Part model, mm, in its own coordinate system. A direction names the side the tool comes from. Round coordinates to 2 decimals unless told otherwise and drop trailing zeros. Order: outer loops, then holes, each group sorted by start corner. A loop starts at its lowest first (then second) coordinate and runs counter-clockwise, first axis right, second up. Notation, with made-up numbers: (74, 46) - (93, 46) arc R19 cw to (93, 62) - close; hole circle Ø1 at (-30.5, 86). An arc over 180 degrees is marked (long way). Return JSON: item names as keys, results as strings. Group by question number.
Item 1: Saw through at A-A on y = 0. List the corners of the cut face in (x, z).
Item 2: Probe probe 1 along Y at (x, z) = (7.5, 36); probe 2 along X at (y, z) = (7, 61); probe 3 along Y at (x, z) = (0, 69). List the from-to ranges inside material, lowest first.
Item 3: Drop flat-ended pins along their axis: pin 1 (5 mm diameter, centred on x = 0, z = 50, fed in from +Y); pin 2 (2.5 mm diameter, centred on y = 0, z = 31.5, fed in from +X). Give the stop position or say it passes through.
Item 4: Two-plate mould, pull along Y, no slides. Class faces 5 (the face through (-2, 2, 0)), 6 (the face through (6, -10, 49)), 7 (the face through (-8, 4, 49)): released by +Y, released by -Y, zero draft, split by the parting line, or undercut.
Item 5: Tool access for faces 1 (the face through (-4, 0, 49)), 2 (the face through (10, 6, 49)), 3 (the face through (0, 4, 49)), 4 (the face through (5, -8, 49)): list every direction of +Z, -Z, +X, -X, +Y, -Y with a clear straight run to the whole face (end or side of a thin tool).
```python
from build123d import *

# Parameters (mm, degrees)
SKETCH2_R           = 2.5
BOSS_EXTRUDE1_DEPTH = 100


with BuildPart() as part:
    # Sketch2 → Boss-Extrude1 (new body)
    with BuildSketch(Plane.XY):
        with BuildLine():
            Line((10, 3.25), (10, 9))
            ThreePointArc((10, 9), (9.707106781, 9.707106781), (9, 10))
            Line((9, 10), (3.25, 10))
            ThreePointArc((3.25, 10), (3.073223305, 9.926776695), (3, 9.75))
            Line((3, 9.75), (3, 8.25))
            ThreePointArc((3, 8.25), (3.073223305, 8.073223305), (3.25, 8))
            Line((3.25, 8), (5.75, 8))
            ThreePointArc((5.75, 8), (5.926776695, 7.926776695), (6, 7.75))
            Line((6, 7.75), (6, 7.164213562))
            ThreePointArc((6, 7.164213562), (5.980969883, 7.068542704), (5.926776695, 6.987436867))
            Line((5.926776695, 6.987436867), (3.085786438, 4.146446609))
            ThreePointArc((3.085786438, 4.146446609), (2.923574763, 4.038060234), (2.732233047, 4))
            Line((2.732233047, 4), (-2.732233047, 4))
            ThreePointArc((-2.732233047, 4), (-2.923574763, 4.038060234), (-3.085786438, 4.146446609))
            Line((-3.085786438, 4.146446609), (-5.926776695, 6.987436867))
            ThreePointArc((-5.926776695, 6.987436867), (-5.980969883, 7.068542704), (-6, 7.164213562))
            Line((-6, 7.164213562), (-6, 7.75))
            ThreePointArc((-6, 7.75), (-5.926776695, 7.926776695), (-5.75, 8))
            Line((-5.75, 8), (-3.25, 8))
            ThreePointArc((-3.25, 8), (-3.073223305, 8.073223305), (-3, 8.25))
            Line((-3, 8.25), (-3, 9.75))
            ThreePointArc((-3, 9.75), (-3.073223305, 9.926776695), (-3.25, 10))
            Line((-3.25, 10), (-9, 10))
            ThreePointArc((-9, 10), (-9.707106781, 9.707106781), (-10, 9))
            Line((-10, 9), (-10, 3.25))
            ThreePointArc((-10, 3.25), (-9.926776695, 3.073223305), (-9.75, 3))
            Line((-9.75, 3), (-8.25, 3))
            ThreePointArc((-8.25, 3), (-8.073223305, 3.073223305), (-8, 3.25))
            Line((-8, 3.25), (-8, 5.75))
            ThreePointArc((-8, 5.75), (-7.926776695, 5.926776695), (-7.75, 6))
            Line((-7.75, 6), (-7.164213562, 6))
            ThreePointArc((-7.164213562, 6), (-7.068542704, 5.980969883), (-6.987436867, 5.926776695))
            Line((-6.987436867, 5.926776695), (-4.146446609, 3.085786438))
            ThreePointArc((-4.146446609, 3.085786438), (-4.038060234, 2.923574763), (-4, 2.732233047))
            Line((-4, 2.732233047), (-4, -2.732233047))
            ThreePointArc((-4, -2.732233047), (-4.038060234, -2.923574763), (-4.146446609, -3.085786438))
            Line((-4.146446609, -3.085786438), (-6.987436867, -5.926776695))
            ThreePointArc((-6.987436867, -5.926776695), (-7.068542704, -5.980969883), (-7.164213562, -6))
            Line((-7.164213562, -6), (-7.75, -6))
            ThreePointArc((-7.75, -6), (-7.926776695, -5.926776695), (-8, -5.75))
            Line((-8, -5.75), (-8, -3.25))
            ThreePointArc((-8, -3.25), (-8.073223305, -3.073223305), (-8.25, -3))
            Line((-8.25, -3), (-9.75, -3))
            ThreePointArc((-9.75, -3), (-9.926776695, -3.073223305), (-10, -3.25))
            Line((-10, -3.25), (-10, -9))
            ThreePointArc((-10, -9), (-9.707106781, -9.707106781), (-9, -10))
            Line((-9, -10), (-3.25, -10))
            ThreePointArc((-3.25, -10), (-3.073223305, -9.926776695), (-3, -9.75))
            Line((-3, -9.75), (-3, -8.25))
            ThreePointArc((-3, -8.25), (-3.073223305, -8.073223305), (-3.25, -8))
            Line((-3.25, -8), (-5.75, -8))
            ThreePointArc((-5.75, -8), (-5.926776695, -7.926776695), (-6, -7.75))
            Line((-6, -7.75), (-6, -7.164213562))
            ThreePointArc((-6, -7.164213562), (-5.980969883, -7.068542704), (-5.926776695, -6.987436867))
            Line((-5.926776695, -6.987436867), (-3.085786438, -4.146446609))
            ThreePointArc((-3.085786438, -4.146446609), (-2.923574763, -4.038060234), (-2.732233047, -4))
            Line((-2.732233047, -4), (2.732233047, -4))
            ThreePointArc((2.732233047, -4), (2.923574763, -4.038060234), (3.085786438, -4.146446609))
            Line((3.085786438, -4.146446609), (5.926776695, -6.987436867))
            ThreePointArc((5.926776695, -6.987436867), (5.980969883, -7.068542704), (6, -7.164213562))
            Line((6, -7.164213562), (6, -7.75))
            ThreePointArc((6, -7.75), (5.926776695, -7.926776695), (5.75, -8))
            Line((5.75, -8), (3.25, -8))
            ThreePointArc((3.25, -8), (3.073223305, -8.073223305), (3, -8.25))
            Line((3, -8.25), (3, -9.75))
            ThreePointArc((3, -9.75), (3.073223305, -9.926776695), (3.25, -10))
            Line((3.25, -10), (9, -10))
            ThreePointArc((9, -10), (9.707106781, -9.707106781), (10, -9))
            Line((10, -9), (10, -3.25))
            ThreePointArc((10, -3.25), (9.926776695, -3.073223305), (9.75, -3))
            Line((9.75, -3), (8.25, -3))
            ThreePointArc((8.25, -3), (8.073223305, -3.073223305), (8, -3.25))
            Line((8, -3.25), (8, -5.75))
            ThreePointArc((8, -5.75), (7.926776695, -5.926776695), (7.75, -6))
            Line((7.75, -6), (7.164213562, -6))
            ThreePointArc((7.164213562, -6), (7.068542704, -5.980969883), (6.987436867, -5.926776695))
            Line((6.987436867, -5.926776695), (4.146446609, -3.085786438))
            ThreePointArc((4.146446609, -3.085786438), (4.038060234, -2.923574763), (4, -2.732233047))
            Line((4, -2.732233047), (4, 2.732233047))
            ThreePointArc((4, 2.732233047), (4.038060234, 2.923574763), (4.146446609, 3.085786438))
            Line((4.146446609, 3.085786438), (6.987436867, 5.926776695))
            ThreePointArc((6.987436867, 5.926776695), (7.068542704, 5.980969883), (7.164213562, 6))
            Line((7.164213562, 6), (7.75, 6))
            ThreePointArc((7.75, 6), (7.926776695, 5.926776695), (8, 5.75))
            Line((8, 5.75), (8, 3.25))
            ThreePointArc((8, 3.25), (8.073223305, 3.073223305), (8.25, 3))
            Line((8.25, 3), (9.75, 3))
            ThreePointArc((9.75, 3), (9.926776695, 3.073223305), (10, 3.25))
        make_face()
        Circle(SKETCH2_R, mode=Mode.SUBTRACT)
    extrude(amount=BOSS_EXTRUDE1_DEPTH)


solid = part.part
```
Filled in:
{
 "1": {"outline": "(-4, 0) - (-2.5, 0) - (-2.5, 100) - (-4, 100) - close; (2.5, 0) - (4, 0) - (4, 100) - (2.5, 100) - close"},
 "2": {"probe 1": "y = -10 to -6, 6 to 10", "probe 2": "x = -10 to -5.94, 5.94 to 10", "probe 3": "y = -4 to -2.5, 2.5 to 4"},
 "3": {"pin 1": "stops at y = 4", "pin 2": "stops at x = 4"},
 "4": {"face 5": "zero draft", "face 6": "released by -Y", "face 7": "undercut"},
 "5": {"face 1": "+Z, -Z, -X", "face 2": "+Z, -Z, +X, +Y, -Y", "face 3": "+Z, -Z, +Y", "face 4": "+Z, -Z"}
}
